The listing builds one solid part. Answer for the finished solid, in the listing's coordinates (mm). A direction names the side the tool comes from. Round coordinates to 2 decimals unless told otherwise and drop trailing zeros. Order: outer loops, then holes, each group sorted by start corner. A loop starts at its lowest first (then second) coordinate and runs counter-clockwise, first axis right, second up. Notation, with made-up numbers: (29.25, 10) - (73.25, 10) arc R25 ccw to (73.25, 35) - close; hole circle Ø8 at (85, 30.5). An arc over 180 degrees is marked (long way). One line per item, written item: value. Start each with the question number.
1. A tool of negligible diameter and unlimited length cuts with its end or side. For faces 1 (the flat face through (0, -17, -10)), 2 (the flat face through (0, 17, -10)), 3 (the flat face through (-2, -22, 12)), from which of +Z, -Z, +X, -X, +Y, -Y can it reach the whole face along a straight path? Write none if from no direction.
2. Section D-D, the plane z = -16 is taken. Give the vertices of the cut face in (x, y).
3. For a pull along X with two mould halves and no side action, classify faces 4 (the cylindrical face through (0.07, 18.52, -11.5)), 5 (the flat face through (-2, 22, 12)), 6 (the cylindrical face through (0.1, -21.5, 7.5)) as released by +X, released by -X, zero draft, split by the parting line, or undercut.
4. Section C-C, the plane z = 1.5 is taken. Give the vertices of the cut face in (x, y).
5. Section B-B, the plane x = 8.75 is taken. Give the vertices of the cut face in (y, z), then the cut area to 3 significant figures.
6. Flat-ended cylindrical pins translate along their axes: P1, Ø3.5, axis at x = 0, z = -9.5, coming from the -Y side; P2, Ø2.5, axis at x = 0, z = -10, coming from the -Y side; P3, Ø4, axis at x = 6.5, z = -15, coming from the +Y side. Find the tip coordinate at first contact, or state that the pin passes through.
7. Straight lines are drawn through the part: line 1 (Y direction, x = -7.5, z = 5); line 2 (Y direction, x = 4.25, z = 13.5); line 3 (X direction, y = 13, z = 10). For each, find the intervals that lie inside material, in ascending order.
8. Section A-A, the plane z = -10 is taken. Give the vertices of the cut face in (x, y).
from build123d import *

# Parameters (mm, degrees)
SKETCH_1_W          = 40
SKETCH_1_H          = 40
EXTRUDE_1_DEPTH     = 10
SKETCH_2_R          = 5
EXTRUDE_2_DEPTH     = 1
SKETCH_3_R          = 2.5
EXTRUDE_3_DEPTH     = 1
SKETCH_4_R          = 10
EXTRUDE_4_DEPTH     = 4
CUT_EXTRUDE_START   = -46
SKETCH_5_R          = 1.25
CUT_EXTRUDE_1_DEPTH = 46
FILLET_1_R          = 2
SKETCH_6_R          = 1.5
CUT_EXTRUDE_2_DEPTH = 3


with BuildPart() as part:
    # 草图1 → 凸台-拉伸1 (new, symmetric)
    with BuildSketch(Plane(origin=(0, 0, 0), x_dir=(0, 0, -1), z_dir=(1, 0, 0))):
        Rectangle(SKETCH_1_W, SKETCH_1_H)
    extrude(amount=EXTRUDE_1_DEPTH, both=True)

    # 草图2 → 凸台-拉伸2 (add)
    with BuildSketch(Plane(origin=(0, 20, 0), x_dir=(1, 0, 0), z_dir=(0, 1, 0))):
        with Locations(Location((0, -10, 0), (0, 0, 90))):
            Circle(SKETCH_2_R)
    extrude_2 = extrude(amount=EXTRUDE_2_DEPTH)

    # 草图3 → 凸台-拉伸3 (add)
    with BuildSketch(Plane(origin=(0, 21, 0), x_dir=(1, 0, 0), z_dir=(0, 1, 0))):
        with Locations(Location((0, -10, 0), (0, 0, 270))):
            Circle(SKETCH_3_R)
    extrude_3 = extrude(amount=EXTRUDE_3_DEPTH)

    # 草图4 → 凸台-拉伸4 (add)
    with BuildSketch(Plane(origin=(0, 22, 0), x_dir=(1, 0, 0), z_dir=(0, 1, 0))):
        with Locations(Location((0, -10, 0), (0, 0, 270))):
            Circle(SKETCH_4_R)
    extrude_4 = extrude(amount=EXTRUDE_4_DEPTH)

    # 草图5 → 切除-拉伸1 (cut)
    with BuildSketch(Plane(origin=(0, 26, 0), x_dir=(1, 0, 0), z_dir=(0, 1, 0)).offset(CUT_EXTRUDE_START)):
        with Locations(Location((0, -10, 0), (0, 0, 270))):
            Circle(SKETCH_5_R)
    cut_extrude_1 = extrude(amount=CUT_EXTRUDE_1_DEPTH, mode=Mode.SUBTRACT)

    # 镜向1: 凸台-拉伸2, 凸台-拉伸3, 凸台-拉伸4, 切除-拉伸1 across plane
    add(extrude_2.mirror(Plane.ZX))
    add(extrude_3.mirror(Plane.ZX))
    add(extrude_4.mirror(Plane.ZX))
    add(cut_extrude_1.mirror(Plane.ZX), mode=Mode.SUBTRACT)

    # 圆角1
    # the kernel refuses this fillet: 2 mm, written as the material it adds along each edge
    with BuildSketch(Plane(origin=(0, 20, 10), x_dir=(0, 0, -1), z_dir=(1, 0, 0))) as fillet_1_piece_1:
        with BuildLine():
            CenterArc((6.732050808, 2), FILLET_1_R, 210, 60)
            Line((6.732050808, 0), (5, 0))
            Line((5, 0), (5, 1))
        make_face()
    revolve(axis=Axis((0, 20, 10), (0, 1, 0)))
    # the kernel refuses this fillet: 2 mm, written as the material it takes off along each edge
    with BuildSketch(Plane(origin=(8, 18, -18), x_dir=(0, 0, -1), z_dir=(0, 1, 0))) as fillet_1_2_piece_1_section:
        Polygon((0, 0), (FILLET_1_R * 1.02, 0), (FILLET_1_R * 1.02, -FILLET_1_R * 1.02), (0, -FILLET_1_R * 1.02), align=None)
    fillet_1_2_piece_1 = extrude(amount=FILLET_1_R * 1.02, mode=Mode.PRIVATE)
    fillet_1_2_piece_1 = fillet_1_2_piece_1 - Plane(origin=(8, 18, -18), x_dir=(-0.7071067811865475, 0, 0.7071067811865475), z_dir=(0, 1, 0)) * Sphere(FILLET_1_R, mode=Mode.PRIVATE)
    add(fillet_1_2_piece_1, mode=Mode.SUBTRACT)
    with BuildSketch(Plane(origin=(8, -18, -18), x_dir=(0, 0, -1), z_dir=(0, -1, 0))) as fillet_1_2_piece_2_section:
        Polygon((0, 0), (FILLET_1_R * 1.02, 0), (FILLET_1_R * 1.02, FILLET_1_R * 1.02), (0, FILLET_1_R * 1.02), align=None)
    fillet_1_2_piece_2 = extrude(amount=FILLET_1_R * 1.02, mode=Mode.PRIVATE)
    fillet_1_2_piece_2 = fillet_1_2_piece_2 - Plane(origin=(8, -18, -18), x_dir=(-0.7071067811865475, 0, 0.7071067811865475), z_dir=(0, -1, 0)) * Sphere(FILLET_1_R, mode=Mode.PRIVATE)
    add(fillet_1_2_piece_2, mode=Mode.SUBTRACT)
    with BuildSketch(Plane(origin=(8, 18, 18), x_dir=(1, 0, 0), z_dir=(0, 1, 0))) as fillet_1_2_piece_3_section:
        Polygon((0, 0), (FILLET_1_R * 1.02, 0), (FILLET_1_R * 1.02, -FILLET_1_R * 1.02), (0, -FILLET_1_R * 1.02), align=None)
    fillet_1_2_piece_3 = extrude(amount=FILLET_1_R * 1.02, mode=Mode.PRIVATE)
    fillet_1_2_piece_3 = fillet_1_2_piece_3 - Plane(origin=(8, 18, 18), x_dir=(-0.7071067811865475, 0, -0.7071067811865475), z_dir=(0, 1, 0)) * Sphere(FILLET_1_R, mode=Mode.PRIVATE)
    add(fillet_1_2_piece_3, mode=Mode.SUBTRACT)
    with BuildSketch(Plane(origin=(8, -18, 18), x_dir=(1, 0, 0), z_dir=(0, -1, 0))) as fillet_1_2_piece_4_section:
        Polygon((0, 0), (FILLET_1_R * 1.02, 0), (FILLET_1_R * 1.02, FILLET_1_R * 1.02), (0, FILLET_1_R * 1.02), align=None)
    fillet_1_2_piece_4 = extrude(amount=FILLET_1_R * 1.02, mode=Mode.PRIVATE)
    fillet_1_2_piece_4 = fillet_1_2_piece_4 - Plane(origin=(8, -18, 18), x_dir=(-0.7071067811865475, 0, -0.7071067811865475), z_dir=(0, -1, 0)) * Sphere(FILLET_1_R, mode=Mode.PRIVATE)
    add(fillet_1_2_piece_4, mode=Mode.SUBTRACT)
    with BuildSketch(Plane(origin=(-8, 18, 18), x_dir=(-1, 0, 0), z_dir=(0, 1, 0))) as fillet_1_2_piece_5_section:
        Polygon((0, 0), (FILLET_1_R * 1.02, 0), (FILLET_1_R * 1.02, FILLET_1_R * 1.02), (0, FILLET_1_R * 1.02), align=None)
    fillet_1_2_piece_5 = extrude(amount=FILLET_1_R * 1.02, mode=Mode.PRIVATE)
    fillet_1_2_piece_5 = fillet_1_2_piece_5 - Plane(origin=(-8, 18, 18), x_dir=(0.7071067811865475, 0, -0.7071067811865475), z_dir=(0, 1, 0)) * Sphere(FILLET_1_R, mode=Mode.PRIVATE)
    add(fillet_1_2_piece_5, mode=Mode.SUBTRACT)
    with BuildSketch(Plane(origin=(-8, 18, -18), x_dir=(0, 0, -1), z_dir=(0, 1, 0))) as fillet_1_2_piece_6_section:
        Polygon((0, 0), (FILLET_1_R * 1.02, 0), (FILLET_1_R * 1.02, FILLET_1_R * 1.02), (0, FILLET_1_R * 1.02), align=None)
    fillet_1_2_piece_6 = extrude(amount=FILLET_1_R * 1.02, mode=Mode.PRIVATE)
    fillet_1_2_piece_6 = fillet_1_2_piece_6 - Plane(origin=(-8, 18, -18), x_dir=(0.7071067811865475, 0, 0.7071067811865475), z_dir=(0, 1, 0)) * Sphere(FILLET_1_R, mode=Mode.PRIVATE)
    add(fillet_1_2_piece_6, mode=Mode.SUBTRACT)
    with BuildSketch(Plane(origin=(-8, -18, -18), x_dir=(0, 0, -1), z_dir=(0, -1, 0))) as fillet_1_2_piece_7_section:
        Polygon((0, 0), (FILLET_1_R * 1.02, 0), (FILLET_1_R * 1.02, -FILLET_1_R * 1.02), (0, -FILLET_1_R * 1.02), align=None)
    fillet_1_2_piece_7 = extrude(amount=FILLET_1_R * 1.02, mode=Mode.PRIVATE)
    fillet_1_2_piece_7 = fillet_1_2_piece_7 - Plane(origin=(-8, -18, -18), x_dir=(0.7071067811865475, 0, 0.7071067811865475), z_dir=(0, -1, 0)) * Sphere(FILLET_1_R, mode=Mode.PRIVATE)
    add(fillet_1_2_piece_7, mode=Mode.SUBTRACT)
    with BuildSketch(Plane(origin=(-8, -18, 18), x_dir=(-1, 0, 0), z_dir=(0, -1, 0))) as fillet_1_2_piece_8_section:
        Polygon((0, 0), (FILLET_1_R * 1.02, 0), (FILLET_1_R * 1.02, -FILLET_1_R * 1.02), (0, -FILLET_1_R * 1.02), align=None)
    fillet_1_2_piece_8 = extrude(amount=FILLET_1_R * 1.02, mode=Mode.PRIVATE)
    fillet_1_2_piece_8 = fillet_1_2_piece_8 - Plane(origin=(-8, -18, 18), x_dir=(0.7071067811865475, 0, -0.7071067811865475), z_dir=(0, -1, 0)) * Sphere(FILLET_1_R, mode=Mode.PRIVATE)
    add(fillet_1_2_piece_8, mode=Mode.SUBTRACT)
    with BuildSketch(Plane(origin=(10, 18, -20), x_dir=(-1, 0, 0), z_dir=(0, -1, 0)), Plane(origin=(-10, 20, 18), x_dir=(0, -1, 0), z_dir=(0, 0, -1)), Plane(origin=(-10, -18, 20), x_dir=(0, 0, -1), z_dir=(0, 1, 0)), Plane(origin=(10, -20, -18), x_dir=(-1, 0, 0), z_dir=(0, 0, 1))) as fillet_1_2_piece_9:
        with BuildLine():
            CenterArc((FILLET_1_R, -FILLET_1_R), FILLET_1_R, 90, 90)
            Line((0, -FILLET_1_R), (0, 0))
            Line((0, 0), (FILLET_1_R, 0))
        make_face()
    extrude(amount=36, mode=Mode.SUBTRACT)
    with BuildSketch(Plane(origin=(10, 20, 18), x_dir=(0, -1, 0), z_dir=(0, 0, -1)), Plane(origin=(10, -18, 20), x_dir=(0, 0, -1), z_dir=(0, 1, 0)), Plane(origin=(-10, 18, -20), x_dir=(1, 0, 0), z_dir=(0, -1, 0)), Plane(origin=(-10, -20, -18), x_dir=(1, 0, 0), z_dir=(0, 0, 1))) as fillet_1_2_piece_10:
        with BuildLine():
            CenterArc((FILLET_1_R, FILLET_1_R), FILLET_1_R, 180, 90)
            Line((0, FILLET_1_R), (0, 0))
            Line((0, 0), (FILLET_1_R, 0))
        make_face()
    extrude(amount=36, mode=Mode.SUBTRACT)
    with BuildSketch(Plane(origin=(8, 20, 20), x_dir=(0, -1, 0), z_dir=(-1, 0, 0)), Plane(origin=(-8, 20, -20), x_dir=(0, -1, 0), z_dir=(1, 0, 0)), Plane(origin=(-8, -20, -20), x_dir=(0, 0, 1), z_dir=(1, 0, 0)), Plane(origin=(8, -20, 20), x_dir=(0, 0, -1), z_dir=(-1, 0, 0))) as fillet_1_2_piece_11:
        with BuildLine():
            CenterArc((FILLET_1_R, -FILLET_1_R), FILLET_1_R, 90, 90)
            Line((0, -FILLET_1_R), (0, 0))
            Line((0, 0), (FILLET_1_R, 0))
        make_face()
    extrude(amount=16, mode=Mode.SUBTRACT)

    # 草图6 → 切除-拉伸2 (cut)
    with BuildSketch(Plane(origin=(0, 20, 0), x_dir=(1, 0, 0), z_dir=(0, 1, 0))):
        with Locations(Location((0, 10, 0), (0, 0, 270))):
            Circle(SKETCH_6_R)
    cut_extrude_2 = extrude(amount=-CUT_EXTRUDE_2_DEPTH, mode=Mode.SUBTRACT)

    # 镜向2: 切除-拉伸2 across plane
    add(cut_extrude_2.mirror(Plane.ZX), mode=Mode.SUBTRACT)


solid = part.part
Answer list:
1. face 1: -Y
1. face 2: +Y
1. face 3: none
2. outline: (-10, -18) arc R2 ccw to (-8, -20) - (8, -20) arc R2 ccw to (10, -18) - (10, 18) arc R2 ccw to (8, 20) - (-8, 20) arc R2 ccw to (-10, 18) - close
3. face 4: undercut
3. face 5: zero draft
3. face 6: split by the parting line
4. outline: (-10, -18) arc R2 ccw to (-8, -20) - (8, -20) arc R2 ccw to (10, -18) - (10, 18) arc R2 ccw to (8, 20) - (-8, 20) arc R2 ccw to (-10, 18) - close; (-5.27, -26) - (5.27, -26) - (5.27, -22) - (-5.27, -22) - close; (-5.27, 22) - (5.27, 22) - (5.27, 26) - (-5.27, 26) - close
5. outline: (-26, 5.16) - (-22, 5.16) - (-22, 14.84) - (-26, 14.84) - close; (-19.85, -18) arc R1.85 ccw to (-18, -19.85) - (18, -19.85) arc R1.85 ccw to (19.85, -18) - (19.85, 18) arc R1.85 ccw to (18, 19.85) - (-18, 19.85) arc R1.85 ccw to (-19.85, 18) - close; (22, 5.16) - (26, 5.16) - (26, 14.84) - (22, 14.84) - close
5. area: 1,650 mm²
6. P1: stops at y = -20
6. P2: stops at y = -17
6. P3: stops at y = 20
7. line 1: y = -26 to -22, -20 to 20, 22 to 26
7. line 2: y = -26 to -22, -20 to 20.42, 22 to 26
7. line 3: x = -10 to -1.25, 1.25 to 10
8. outline: (-10, -18) arc R2 ccw to (-8, -20) - (-1.5, -20) - (-1.5, -17) - (1.5, -17) - (1.5, -20) - (8, -20) arc R2 ccw to (10, -18) - (10, 18) arc R2 ccw to (8, 20) - (1.5, 20) - (1.5, 17) - (-1.5, 17) - (-1.5, 20) - (-8, 20) arc R2 ccw to (-10, 18) - close
